from build123d import *

# Parameters (mm, degrees)
BOSS_EXTRUDE2_DEPTH     = 20
SKETCH1_7_W             = 270
SKETCH1_7_H             = 40
BOSS_EXTRUDE3_DEPTH     = 40
SKETCH1_9_W             = 30
SKETCH1_9_H             = 80
CUT_EXTRUDE4_DEPTH      = 41
CUT_EXTRUDE4_DEPTH_BACK = 1


with BuildPart() as part:
    # Sketch1 → Boss-Extrude2 (new body)
    with BuildSketch(Plane(origin=(0, 0, 0), x_dir=(1, 0, 0), z_dir=(0, 1, 0))):
        Polygon((0, 0), (270, 0), (280, 280), (-10, 280), align=None)
    extrude(amount=BOSS_EXTRUDE2_DEPTH)

    # Sketch1_7 → Boss-Extrude3 (add)
    with BuildSketch(Plane(origin=(0, 0, 0), x_dir=(1, 0, 0), z_dir=(0, 1, 0))):
        with Locations((135, 50)):
            Rectangle(SKETCH1_7_W, SKETCH1_7_H)
    extrude(amount=BOSS_EXTRUDE3_DEPTH)

    # Sketch1_9 → Cut-Extrude4 (cut, two sides)
    with BuildSketch(Plane(origin=(0, 0, 0), x_dir=(1, 0, 0), z_dir=(0, 1, 0))) as cut_extrude4_sk:
        with Locations((135, 40)):
            Rectangle(SKETCH1_9_W, SKETCH1_9_H)
    extrude(amount=CUT_EXTRUDE4_DEPTH, mode=Mode.SUBTRACT)
    extrude(cut_extrude4_sk.sketch, amount=-CUT_EXTRUDE4_DEPTH_BACK, mode=Mode.SUBTRACT)


solid = part.part
Source: CAD feature listing. Evaluate the final solid. Frame: model axes, mm. A direction names the side the tool comes from. Coordinates: 2 decimals unless noted, no trailing zeros. Loops run counter-clockwise (first coordinate to the right, second up) from the corner with the lowest first, then second, coordinate; pieces in that order, holes last. Notation, with made-up numbers: (-5.5, 79.25) - (8.5, 79.25) arc R25 ccw to (8.5, 116.25) - close; hole circle Ø4 at (82, -27). An arc over 180 degrees is marked (long way). One line per item, written item: value. Start each with the question number.
1. Section A-A (y = 24). Return the cut outline in (x, z).
2. Section B-B (x = 101.5). Return the cut outline in (y, z).
3. Section C-C (z = -48.5). Return the cut outline in (x, y).
4. Contact query for flat-ended pins moving along their axis: P1, Ø10, axis at x = 210, y = 26.5, coming from the -Z side; P2, Ø12, axis at y = 13.5, z = -56.5, coming from the +X side; P3, Ø6, axis at x = 131, y = 5.5, coming from the +Z side; P4, Ø6, axis at x = 164.5, z = -251.5, coming from the -Y side. Output: stop coordinate, or through.
5. Set-up query: faces 1 (the flat face through (120, 15, -39)), 2 (the flat face through (0, 30, -50)), 3 (the flat face through (209, 30, -70)). Return all of +Z, -Z, +X, -X, +Y, -Y with unobstructed straight access to the full face (end or side cutting, diameter ignored); none if empty.
6. Ray query, L1, parallel to Z at x = 33.5, y = 25.5; L2, parallel to Z at x = 121, y = 3; L3, parallel to Y at x = 109.5, z = -22. Return the intervals inside material, ascending.
7. Section D-D (y = 4.5). Return the cut outline in (x, z), and give its area (3 significant figures).
Verdict:
1. outline: (0, -70) - (120, -70) - (120, -30) - (0, -30) - close; (150, -70) - (270, -70) - (270, -30) - (150, -30) - close
2. outline: (0, -280) - (20, -280) - (20, -70) - (40, -70) - (40, -30) - (20, -30) - (20, 0) - (0, 0) - close
3. outline: (-1.73, 0) - (120, 0) - (120, 40) - (0, 40) - (0, 20) - (-1.73, 20) - close; (150, 0) - (271.73, 0) - (271.73, 20) - (270, 20) - (270, 40) - (150, 40) - close
4. P1: stops at z = -70
4. P2: stops at x = 272.23
4. P3: stops at z = -80
4. P4: stops at y = 0
5. face 1: +Z, +Y, -Y
5. face 2: +Z, -Z, -X, +Y
5. face 3: -Z, +X, -X, +Y
6. L1: z = -70 to -30
6. L2: z = -280 to -80
6. L3: y = 0 to 20
7. outline: (-10, -280) - (280, -280) - (270, 0) - (150, 0) - (150, -80) - (120, -80) - (120, 0) - (0, 0) - close
7. area: 76,000 mm2
